```python
from build123d import *

# Parameters (mm, degrees)
EXTRUDE_1_DEPTH     = 2.4
CUT_EXTRUDE_2_DEPTH = 1
SKETCH_3_R          = 1.5
CUT_EXTRUDE_3_DEPTH = 54.793679926


with BuildPart() as part:
    # 스케치1 → 보스-돌출1 (new body)
    with BuildSketch(Plane(origin=(0, 0, 0), x_dir=(1, 0, 0), z_dir=(0, 1, 0))):
        with BuildLine():
            ThreePointArc((33, -33), (0, -38), (-33, -33))
            ThreePointArc((-33, -33), (-38, 0), (-33, 33))
            ThreePointArc((-33, 33), (0, 38), (33, 33))
            ThreePointArc((33, 33), (38, 0), (33, -33))
        make_face()
        with BuildLine():
            Line((-22.5, 30.81662479), (-22.5, 31.616712956))
            ThreePointArc((-22.5, 31.616712956), (-11.312935706, 33.402516289), (0, 34))
            ThreePointArc((0, 34), (11.312935706, 33.402516289), (22.5, 31.616712956))
            Line((22.5, 31.616712956), (22.5, 30.81662479))
            ThreePointArc((22.5, 30.81662479), (23.257359313, 23.257359313), (30.81662479, 22.5))
            Line((30.81662479, 22.5), (31.616712956, 22.5))
            ThreePointArc((31.616712956, 22.5), (33.402516289, 11.312935706), (34, 0))
            ThreePointArc((34, 0), (33.402516289, -11.312935706), (31.616712956, -22.5))
            Line((31.616712956, -22.5), (30.81662479, -22.5))
            ThreePointArc((30.81662479, -22.5), (23.257359313, -23.257359313), (22.5, -30.81662479))
            Line((22.5, -30.81662479), (22.5, -31.616712956))
            ThreePointArc((22.5, -31.616712956), (11.312935706, -33.402516289), (0, -34))
            ThreePointArc((0, -34), (-11.312935706, -33.402516289), (-22.5, -31.616712956))
            Line((-22.5, -31.616712956), (-22.5, -30.81662479))
            ThreePointArc((-22.5, -30.81662479), (-23.257359313, -23.257359313), (-30.81662479, -22.5))
            Line((-30.81662479, -22.5), (-31.616712956, -22.5))
            ThreePointArc((-31.616712956, -22.5), (-33.402516289, -11.312935706), (-34, 0))
            ThreePointArc((-34, 0), (-33.402516289, 11.312935706), (-31.616712956, 22.5))
            Line((-31.616712956, 22.5), (-30.81662479, 22.5))
            ThreePointArc((-30.81662479, 22.5), (-23.257359313, 23.257359313), (-22.5, 30.81662479))
        make_face(mode=Mode.SUBTRACT)
    extrude(amount=EXTRUDE_1_DEPTH)

    # 스케치2 → 컷-돌출2 (cut)
    with BuildSketch(Plane(origin=(0, 0, 0), x_dir=(1, 0, 0), z_dir=(0, 1, 0))):
        with BuildLine():
            Line((-24.5, 30.145751311), (-24.5, 33.220870434))
            ThreePointArc((-24.5, 33.220870434), (-12.328534192, 35.302655242), (0, 35.999543016))
            ThreePointArc((0, 35.999543016), (12.328534192, 35.302655242), (24.5, 33.220870434))
            Line((24.5, 33.220870434), (24.5, 30.145751311))
            ThreePointArc((24.5, 30.145751311), (24.671572875, 24.671572875), (30.145751311, 24.5))
            Line((30.145751311, 24.5), (33.220870434, 24.5))
            ThreePointArc((33.220870434, 24.5), (35.302655242, 12.328534192), (35.999543016, 0))
            ThreePointArc((35.999543016, 0), (35.302655242, -12.328534192), (33.220870434, -24.5))
            Line((33.220870434, -24.5), (30.145751311, -24.5))
            ThreePointArc((30.145751311, -24.5), (24.671572875, -24.671572875), (24.5, -30.145751311))
            Line((24.5, -30.145751311), (24.5, -33.220870434))
            ThreePointArc((24.5, -33.220870434), (12.328534192, -35.302655242), (0, -35.999543016))
            ThreePointArc((0, -35.999543016), (-12.328534192, -35.302655242), (-24.5, -33.220870434))
            Line((-24.5, -33.220870434), (-24.5, -30.145751311))
            ThreePointArc((-24.5, -30.145751311), (-24.671572875, -24.671572875), (-30.145751311, -24.5))
            Line((-30.145751311, -24.5), (-33.220870434, -24.5))
            ThreePointArc((-33.220870434, -24.5), (-35.302655242, -12.328534192), (-35.999543016, 0))
            ThreePointArc((-35.999543016, 0), (-35.302655242, 12.328534192), (-33.220870434, 24.5))
            Line((-33.220870434, 24.5), (-30.145751311, 24.5))
            ThreePointArc((-30.145751311, 24.5), (-24.671572875, 24.671572875), (-24.5, 30.145751311))
        make_face()
        with BuildLine():
            Line((-23.5, 30.5), (-23.5, 32.421599525))
            ThreePointArc((-23.5, 32.421599525), (-11.820488491, 34.353129782), (0, 34.999543016))
            ThreePointArc((0, 34.999543016), (11.820488491, 34.353129782), (23.5, 32.421599525))
            Line((23.5, 32.421599525), (23.5, 30.5))
            ThreePointArc((23.5, 30.5), (23.964466094, 23.964466094), (30.5, 23.5))
            Line((30.5, 23.5), (32.421599525, 23.5))
            ThreePointArc((32.421599525, 23.5), (34.353129782, 11.820488491), (34.999543016, 0))
            ThreePointArc((34.999543016, 0), (34.353129782, -11.820488491), (32.421599525, -23.5))
            Line((32.421599525, -23.5), (30.5, -23.5))
            ThreePointArc((30.5, -23.5), (23.964466094, -23.964466094), (23.5, -30.5))
            Line((23.5, -30.5), (23.5, -32.421599525))
            ThreePointArc((23.5, -32.421599525), (11.820488491, -34.353129782), (0, -34.999543016))
            ThreePointArc((0, -34.999543016), (-11.820488491, -34.353129782), (-23.5, -32.421599525))
            Line((-23.5, -32.421599525), (-23.5, -30.5))
            ThreePointArc((-23.5, -30.5), (-23.964466094, -23.964466094), (-30.5, -23.5))
            Line((-30.5, -23.5), (-32.421599525, -23.5))
            ThreePointArc((-32.421599525, -23.5), (-34.353129782, -11.820488491), (-34.999543016, 0))
            ThreePointArc((-34.999543016, 0), (-34.353129782, 11.820488491), (-32.421599525, 23.5))
            Line((-32.421599525, 23.5), (-30.5, 23.5))
            ThreePointArc((-30.5, 23.5), (-23.964466094, 23.964466094), (-23.5, 30.5))
        make_face(mode=Mode.SUBTRACT)
    extrude(amount=CUT_EXTRUDE_2_DEPTH, mode=Mode.SUBTRACT)

    # 스케치3 → 컷-돌출3 (cut, through all)
    with BuildSketch(Plane(origin=(0, 0, 0), x_dir=(1, 0, 0), z_dir=(0, 1, 0))):
        with Locations(Location((-27.5, 27.5, 0), (0, 0, 270))):
            Circle(SKETCH_3_R)
        with Locations(Location((27.5, 27.5, 0), (0, 0, 270))):
            Circle(SKETCH_3_R)
        with Locations(Location((27.5, -27.5, 0), (0, 0, 270))):
            Circle(SKETCH_3_R)
        with Locations(Location((-27.5, -27.5, 0), (0, 0, 270))):
            Circle(SKETCH_3_R)
    extrude(amount=CUT_EXTRUDE_3_DEPTH, mode=Mode.SUBTRACT)


solid = part.part
```
Source: CAD feature listing. Evaluate the final solid. Frame: model axes, mm. A direction names the side the tool comes from. Round coordinates to 2 decimals unless told otherwise and drop trailing zeros. Order: outer loops, then holes, each group sorted by start corner. A loop starts at its lowest first (then second) coordinate and runs counter-clockwise, first axis right, second up. Notation, with made-up numbers: (-17, 27) -> (-10, 27) arc R14 cw to (-10, 51) -> close; hole circle Ø1 at (32, 59.5). An arc over 180 degrees is marked (long way). Use CSV: the item, a comma, the result in double quotes.
(1) Section D-D on x = -27.5. Return the cut outline in (y, z).
Report:
outline,"(0, -34.55) -> (2.4, -34.55) -> (2.4, -29) -> (0, -29) -> close; (0, -26) -> (2.4, -26) -> (2.4, -21.5) -> (0, -21.5) -> (0, -22.5) -> (1, -22.5) -> (1, -23.5) -> (0, -23.5) -> close; (0, 21.5) -> (2.4, 21.5) -> (2.4, 26) -> (0, 26) -> (0, 23.5) -> (1, 23.5) -> (1, 22.5) -> (0, 22.5) -> close; (0, 29) -> (2.4, 29) -> (2.4, 34.55) -> (0, 34.55) -> close"
(2) First-contact query: pin 1 Ø0.8 at (x, y) = (32, 0.5) entering from +Z; pin 2 Ø1.1 at (y, z) = (0.5, -32.5) entering from +X; pin 3 Ø0.6 at (x, y) = (-31.5, 1.5) entering from +Z. Flat tips, straight axial feed; report the tip coordinate or a pass-through.
Report:
pin 1,"z = 33.42"
pin 2,"x = 33.32"
pin 3,"z = 33.54"
(3) Ray query, L1, parallel to Z at x = -1, y = 2.1; L2, parallel to Z at x = -27.5, y = 0.75; L3, parallel to Z at x = 27.5, y = 1.65. Return the intervals inside material, ascending.
Report:
L1,"-38 to -34, 34 to 38"
L2,"-34.55 to -29, -26 to -23.5, -22.5 to -21.5, 21.5 to 22.5, 23.5 to 26, 29 to 34.55"
L3,"-34.55 to -29, -26 to -21.5, 21.5 to 26, 29 to 34.55"
(4) Section C-C on z = 27.5. Return the cut outline in (x, y).
Report:
outline,"(-34.55, 0) -> (-29, 0) -> (-29, 2.4) -> (-34.55, 2.4) -> close; (-26, 0) -> (-23.5, 0) -> (-23.5, 1) -> (-22.5, 1) -> (-22.5, 0) -> (-21.5, 0) -> (-21.5, 2.4) -> (-26, 2.4) -> close; (21.5, 0) -> (22.5, 0) -> (22.5, 1) -> (23.5, 1) -> (23.5, 0) -> (26, 0) -> (26, 2.4) -> (21.5, 2.4) -> close; (29, 0) -> (34.55, 0) -> (34.55, 2.4) -> (29, 2.4) -> close"
(5) Section B-B on x = 19.5. Return the cut outline in (y, z).
Report:
outline,"(0, -36.28) -> (2.4, -36.28) -> (2.4, -32.21) -> (0, -32.21) -> (0, -33.23) -> (1, -33.23) -> (1, -34.25) -> (0, -34.25) -> close; (0, 32.21) -> (2.4, 32.21) -> (2.4, 36.28) -> (0, 36.28) -> (0, 34.25) -> (1, 34.25) -> (1, 33.23) -> (0, 33.23) -> close"
(6) Access query for faces 1 (the face through (24.2, 1, -24.2)), 2 (the face through (28.51, 1.18, -28.61)). Directions: +Z, -Z, +X, -X, +Y, -Y. A direction counts if a zero-diameter tool reaches every point of the face in a straight line with its end or side. Return the directions, or none.
Report:
face 1,"-Y"
face 2,"+Y, -Y"
(7) Pull-direction query (X, two-part tool) for faces 3 (the face through (0, 1, 38)), 4 (the face through (24.04, 0.49, 23.89)), 5 (the face through (-26.49, 1.18, -28.61)), 6 (the face through (6, 2.4, -34)); classes: +X half, -X half, draft (parallel to the pull), parting line (faces both ways), or undercut.
Report:
face 3,"parting line"
face 4,"undercut"
face 5,"undercut"
face 6,"draft"
(8) Section A-A on y = 1.5. Return the cut outline in (x, z).
Report:
outline,"(-33, -33) arc R111.4 ccw to (33, -33) arc R111.4 ccw to (33, 33) arc R111.4 ccw to (-33, 33) arc R111.4 ccw to start; hole (-31.62, -22.5) -> (-30.82, -22.5) arc R6 cw to (-22.5, -30.82) -> (-22.5, -31.62) arc R107.4 ccw to (22.5, -31.62) -> (22.5, -30.82) arc R6 cw to (30.82, -22.5) -> (31.62, -22.5) arc R107.4 ccw to (31.62, 22.5) -> (30.82, 22.5) arc R6 cw to (22.5, 30.82) -> (22.5, 31.62) arc R107.4 ccw to (-22.5, 31.62) -> (-22.5, 30.82) arc R6 cw to (-30.82, 22.5) -> (-31.62, 22.5) arc R107.4 ccw to start; hole circle Ø3 at (-27.5, -27.5); hole circle Ø3 at (-27.5, 27.5); hole circle Ø3 at (27.5, -27.5); hole circle Ø3 at (27.5, 27.5)"
